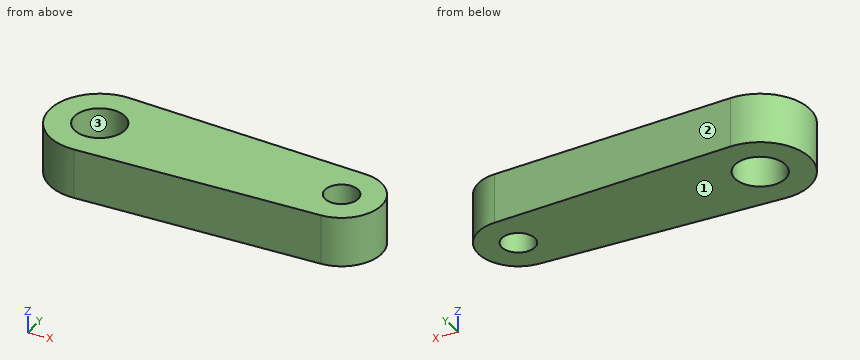
Autodesk Inventor part; units mm, degrees
ref_plane "YZ Plane" through (0, 0, 0) normal (1, 0, 0) x (0, 1, 0)
ref_plane "XZ Plane" through (0, 0, 0) normal (0, 1, 0) x (-1, 0, 0)
ref_plane "XY Plane" through (0, 0, 0) normal (0, 0, 1) x (1, 0, 0)
sketch "Skizze1" plane through (0, 0, 0) normal (0, 0, 1) x (1, 0, 0)
  arc A0 (10.4173, 10) -> (10.4173, -10) centre (10.0084, 0) ccw
  line L0 (10.4173, 10) -> (59.3205, 8)
  line L1 (10.4173, -10) -> (59.3205, -8)
  arc A1 (59.3205, -8) -> (59.3205, 8) centre (58.9933, 0) ccw
  point P0 (0, 0)
  point P1 (67, 0)
  point P2 (0, 0)
  dimension "d0" = 20
  dimension "d1" = 16
  dimension "d2" = 67
extrude "Extrusion1" add sketch "Skizze1" along normal blind 10
sketch "Skizze2" plane through (0, 0, 10) normal (0, 0, 1) x (1, 0, 0)
  arc A0 (10.4173, 10) -> (10.4173, -10) centre (10.0084, 0) ccw
  point P0 (0, 0)
hole "Bohrung1" at (10.0084, 0, 10) direction (0, 0, -1) diameter 10.106 end through all
sketch "Skizze3" plane through (0, 0, 10) normal (0, 0, 1) x (1, 0, 0)
  arc A0 (59.3205, -8) -> (59.3205, 8) centre (58.9933, 0) ccw
  point P0 (0, 0)
hole "Bohrung2" at (58.9933, 0, 10) direction (0, 0, -1) diameter 6.647 end through all
properties part number "Kurbelarm" material "Stahl, galvanisiert"
Could you check a few things on this model? Use its own coordinates, in mm. Face numbers are marked on the shaded views. Coordinates: 2 decimals unless noted, no trailing zeros. Order: outer loops, then holes, each group sorted by start corner. A loop starts at its lowest first (then second) coordinate and runs counter-clockwise, first axis right, second up. Notation, with made-up numbers: M 80,-10.75 L 108,-10.75 A7 ccw 108,-1.75 Z; hole C 30.5,24 d8. An arc over 180 degrees is marked long. Use one line per item in the form item = value. Start each with the question number.
1. Suppose I cut it at C-C on y = -2.5. Write out the boundary of the cut face in (x, z), then the cut area to 3 significant figures.
2. We'd pull the mould along X, two halves only. Please class the marked faces 1, 2 and 3: +X half, -X half, draft (parallel to the pull), parting line (faces both ways), or undercut.
3. Suppose I cut it at D-D on x = 34. Write out the boundary of the cut face in (y, z).
4. For pin 1 (12 mm diameter, centred on x = 40, y = -3.5, fed in from -Z); pin 2 (4 mm diameter, centred on x = 36, z = 4.5, fed in from -Y); pin 3 (3 mm diameter, centred on y = -6, z = 5.5, fed in from -X); pin 4 (5 mm diameter, centred on y = 7.5, z = 9, fed in from -X), each with a flat end and sliding along its axis, tell me the tip position at first contact or that it passes through.
5. Suppose I cut it at B-B on z = 1.25. Write out the boundary of the cut face in (x, y), then the cut area to 3 significant figures.
6. Suppose I cut it at A-A on y = 0. Write out the boundary of the cut face in (x, z).
7. Please list where these lines run through material, in increasing order: line 1 (X direction, y = -1.75, z = 7.75); line 2 (X direction, y = 1.25, z = 6); line 3 (Y direction, x = 10, z = 9).
Geometry says:
q1.outline = M 0.32,0 L 5.62,0 L 5.62,10 L 0.32,10 Z; M 14.4,0 L 56.8,0 L 56.8,10 L 14.4,10 Z; M 61.18,0 L 66.6,0 L 66.6,10 L 61.18,10 Z
q1.area = 531 mm^2
q2.face_1 = draft
q2.face_2 = +X half
q2.face_3 = undercut
q3.outline = M -9.04,0 L 9.04,0 L 9.04,10 L -9.04,10 Z
q4.pin_1 = 0
q4.pin_2 = -9.04
q4.pin_3 = 1.07
q4.pin_4 = 1.34
q5.outline = M 10.42,-10 L 59.32,-8 A8.01 ccw 59.32,8 L 10.42,10 A10.01 ccw long Z; hole C 10.01,0 d10.11; hole C 58.99,0 d6.65
q5.area = 1,030 mm^2
q6.outline = M 0,0 L 4.96,0 L 4.96,10 L 0,10 Z; M 15.06,0 L 55.67,0 L 55.67,10 L 15.06,10 Z; M 62.32,0 L 67,0 L 67,10 L 62.32,10 Z
q7.line_1 = 0.15 to 5.27, 14.75 to 56.17, 61.82 to 66.81
q7.line_2 = 0.08 to 5.11, 14.9 to 55.91, 62.07 to 66.9
q7.line_3 = -10.01 to -5.05, 5.05 to 10.01
